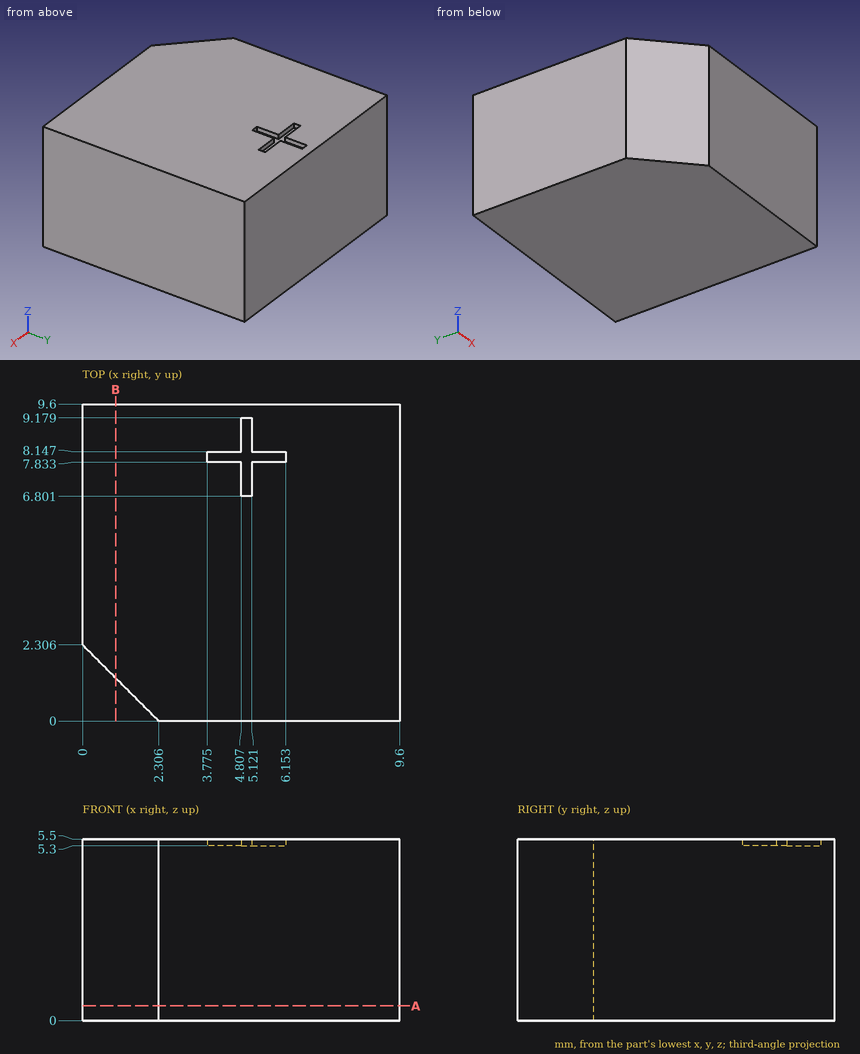
Geometry: see drawing. Coordinates: mm, zero at the bounding-box minimum. Round coordinates to 2 decimals unless told otherwise and drop trailing zeros. Order: outer loops, then holes, each group sorted by start corner. A loop starts at its lowest first (then second) coordinate and runs counter-clockwise, first axis right, second up. Notation, with made-up numbers: (-33, 34) -> (12, 34) arc R9 cw to (12, 47) -> close; hole circle Ø2 at (-39, 8). An arc over 180 degrees is marked (long way). Write each question's results on one line, items separated by ' | '.
Q1. Section query A-A (z = 0.45). Output: boundary loops of the cut face in (x, y), and give its area (3 significant figures).
Response values:
outline: (0, 2.31) -> (2.31, 0) -> (9.6, 0) -> (9.6, 9.6) -> (0, 9.6) -> close | area: 89.5 mm²
Q2. Ray query, line 1 along Y through (x, z) = (1.25, 1.75) (1 decimal); line 2 along Y through (x, z) = (1, 0.3) (1 decimal). Return the intervals inside material, ascending.
Response values:
line 1: 1.1 to 9.6 | line 2: 1.3 to 9.6
Q3. Pin query (flat end, axial travel): pin 1 Ø0.7 at (x, y) = (5, 8.5) entering from +Z. Return the tip coordinate at first contact, or that it passes through.
Response values:
pin 1: z = 5.5
Q4. Section query B-B (x = 1). Output: boundary loops of the cut face in (y, z), and give its area (3 significant figures).
Response values:
outline: (1.31, 0) -> (9.6, 0) -> (9.6, 5.5) -> (1.31, 5.5) -> close | area: 45.6 mm²
